Could you check a few things on this model? Use its own coordinates, in mm. Face numbers are marked on the shaded views. A direction names the side the tool comes from. Round coordinates to 2 decimals unless told otherwise and drop trailing zeros. Loops run counter-clockwise (first coordinate to the right, second up) from the corner with the lowest first, then second, coordinate; pieces in that order, holes last.
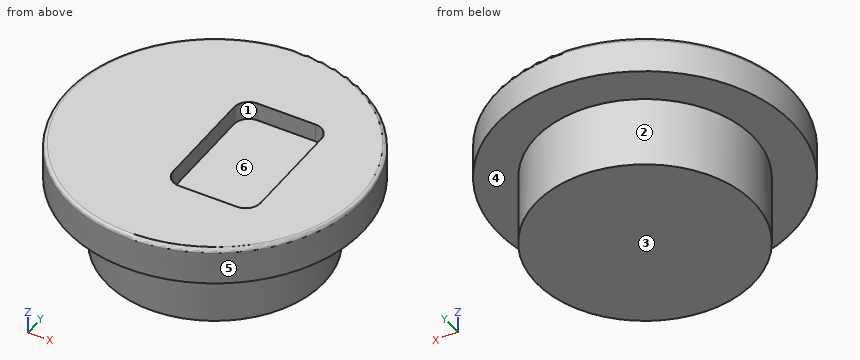
from build123d import *

# Parameters (mm, degrees)
SKETCH_R     = 40
PAD_DEPTH    = 10
FILLET_R     = 1
SKETCH001_R  = 29.5
PAD001_DEPTH = 19.3
POCKET_DEPTH = 5


with BuildPart() as part:
    # Sketch → Pad (new body)
    with BuildSketch(Plane.XY):
        Circle(SKETCH_R)
    extrude(amount=PAD_DEPTH)

    # Fillet
    fillet_edges = [part.edges().sort_by_distance(p)[0] for p in [
        (-40, 0, 10),
    ]]
    fillet(fillet_edges, radius=FILLET_R)

    # Sketch001 → Pad001 (new body)
    with BuildSketch(Plane(origin=(0, 0, 0), x_dir=(1, 0, 0), z_dir=(0, 0, -1))):
        Circle(SKETCH001_R)
    extrude(amount=PAD001_DEPTH)

    # Sketch002 → Pocket (cut)
    with BuildSketch(Plane.XY.offset(10)):
        with BuildLine():
            Line((0.9, 18), (16.468855, 18))
            ThreePointArc((20.468855, 14), (19.297282, 16.828427), (16.468855, 18))
            Line((20.468855, 14), (20.468855, -14))
            ThreePointArc((16.468855, -18), (19.297282, -16.828427), (20.468855, -14))
            Line((16.468855, -18), (0.9, -18))
            ThreePointArc((-3.1, -14), (-1.928427, -16.828427), (0.9, -18))
            Line((-3.1, -14), (-3.1, 14))
            ThreePointArc((0.9, 18), (-1.928427, 16.828427), (-3.1, 14))
        make_face()
    extrude(amount=-POCKET_DEPTH, mode=Mode.SUBTRACT)


solid = part.part
Item 1: If we section it at A-A, the plane y = 0: Please give me the cut outline in (x, z).
Results list:
outline: (-40, 0) - (-29.5, 0) - (-29.5, -19.3) - (29.5, -19.3) - (29.5, 0) - (40, 0) - (40, 9) arc R1 ccw to (39, 10) - (20.47, 10) - (20.47, 5) - (-3.1, 5) - (-3.1, 10) - (-39, 10) arc R1 ccw to (-40, 9) - close
Item 2: If I drill on line 1 along Z through (x, y) = (-10, -36); line 2 along Z through (x, y) = (16, 12); line 3 along Y through (x, z) = (6.5, -5.5), over which ranges is the centre line in solid material (lowest first)?
Results list:
line 1: z = 0 to 10
line 2: z = -19.3 to 5
line 3: y = -28.77 to 28.77
Item 3: If we section it at B-B, the plane z = -4.75: Please give me the cut outline in (x, y).
Results list:
outline: circle Ø59 at (0, 0)
Item 4: Will these pins go through, and if not, where does the flat tip stop? pin 1 (12 mm diameter, centred on y = 3, z = -14, fed in from +X); pin 2 (1 mm diameter, centred on y = -28, z = 2, fed in from -X); pin 3 (12 mm diameter, centred on y = 30.5, z = 4, fed in from +X).
Results list:
pin 1: stops at x = 29.5
pin 2: stops at x = -29.05
pin 3: stops at x = 31.62
Item 5: For the marked faces 1, 2 and 3, which set-ups out of +Z, -Z, +X, -X, +Y, -Y let a thin tool reach every point of the face, with its end or its side?
Results list:
face 1: +Z
face 2: -Z
face 3: -Z, +X, -X, +Y, -Y
Item 6: We'd pull the mould along X, two halves only. Please class the marked faces 4, 5 and 6: released by +X, released by -X, zero draft, split by the parting line, or undercut.
Results list:
face 4: zero draft
face 5: split by the parting line
face 6: undercut
